Geometry check sheet. Reference: the model listing, model coordinates, mm. Face numbers are marked on the shaded views. Give positions to 0.01 mm unless a question says otherwise; leave off trailing zeros. Write each loop counter-clockwise with the first axis right and the second up, starting at its lowest first coordinate (ties: lowest second). Pieces come first, ordered by that corner, then holes. Notation, with made-up numbers: (-24.5, 32.25) -> (9.5, 32.25) arc R29 cw to (9.5, 71.25) -> close; hole circle Ø9 at (44.5, 72). An arc over 180 degrees is marked (long way). Use a Markdown table: item, result. Add a question column.
Autodesk Inventor part; units mm, degrees
ref_plane "YZ Plane" through (0, 0, 0) normal (1, 0, 0) x (0, 1, 0)
ref_plane "XZ Plane" through (0, 0, 0) normal (0, 1, 0) x (-1, 0, 0)
ref_plane "XY Plane" through (0, 0, 0) normal (0, 0, 1) x (1, 0, 0)
sketch "スケッチ1" plane through (0, 0, 0) normal (0, 0, 1) x (1, 0, 0)
  line L0 (-101.5, 48) -> (108.5, 48)
  circle A0 centre (111.885, -19) radius 4
  circle A1 centre (171.8807, -19.7195) radius 4
  circle A2 centre (111.885, -19) radius 7
  circle A3 centre (171.8807, -19.7195) radius 7
  line L1 (171.8807, -19.7195) -> (111.885, -19) construction
  line L2 (171.9647, -12.72) -> (111.969, -12.0005)
  line L3 (111.8011, -25.9995) -> (171.7968, -26.719)
  arc A4 (171.7968, -26.719) -> (171.9647, -12.72) centre (171.8807, -19.7195) ccw
  arc A5 (111.969, -12.0005) -> (111.8011, -25.9995) centre (111.885, -19) ccw
  line L4 (173.7961, -12.9866) -> (250.1906, -34.7195)
  circle A6 centre (241.9819, -63.5746) radius 30
  line L5 (268.18, -78.1916) -> (221.9512, -41.2414)
  line L6 (221.9512, -41.2414) -> (169.9654, -26.4523)
  line L7 (271.9819, -113.1361) -> (271.9819, -54.8199)
  line L8 (111.885, -19) -> (111.885, 41) construction
  line L9 (118.885, -19) -> (118.885, 41)
  line L10 (104.885, 41) -> (104.885, -19)
  arc A7 (104.885, -19) -> (118.885, -19) centre (111.885, -19) ccw
  arc A8 (118.885, 41) -> (104.885, 41) centre (111.885, 41) ccw
  circle A9 centre (29.4318, 47.238) radius 30
  line L11 (113.3193, 34.1485) -> (35.5787, 17.8745)
  line L12 (-0.5585, 48) -> (57.5489, 36.7771)
  line L13 (57.5489, 36.7771) -> (110.4508, 47.8515)
  circle A10 centre (113.5, -20) radius 68
  line L14 (321.9635, -82.9551) -> (60.2705, 100.2843)
  line L15 (259.1892, -39) -> (111.885, -19)
  arc A11 (93.5924, -27.1048) -> (135.371, -5.9244) centre (95.0604, 21.7941) ccw
  arc A12 (135.371, -5.9244) -> (135.8476, -3.6716) centre (132.899, -4.2246) ccw
  arc A13 (135.8476, -3.6716) -> (83.1833, 18.5565) centre (102.1579, -9.9896) ccw
  line L16 (111.885, -19) -> (112.6892, 40.9946) construction
  line L17 (118.8844, -19.0938) -> (119.6886, 40.9008)
  line L18 (105.6898, 41.0884) -> (104.8857, -18.9062)
  arc A14 (104.8857, -18.9062) -> (118.8844, -19.0938) centre (111.885, -19) ccw
  arc A15 (119.6886, 40.9008) -> (105.6898, 41.0884) centre (112.6892, 40.9946) ccw
  line L19 (164.9949, 48) -> (164.9949, 26)
  line L20 (164.9949, 26) -> (327.4949, -102)
  circle A16 centre (116.2926, -40) radius 68
  circle A17 centre (-98.885, 0) radius 67.5
  line L21 (321.3633, -8.501) -> (-152.6681, 78.4982)
  line L22 (104.8897, -3) -> (104.8897, 0)
  line L23 (104.8897, -3) -> (72.0656, -3)
  line L24 (72.0656, 0) -> (104.8897, 0)
  circle A18 centre (83.3769, -17.5) radius 13.85
  line L25 (178.7705, -28.9572) -> (174.2123, -32.8589)
  line L26 (174.2123, -32.8589) -> (164.8807, -30.2042)
  line L27 (164.8807, -30.2042) -> (164.8807, -19.7195)
  line L28 (169.9654, -26.4523) -> (168.5972, -31.2615)
  line L29 (168.5972, -31.2615) -> (164.8807, -26.636)
  line L30 (178.8802, -19.8034) -> (178.6547, -38.6089)
  line L31 (165.0125, -21.0715) -> (158.1724, 13.6763)
  circle A19 centre (171.8807, -19.7195) radius 7.5
  point P0 (0, 0)
  point P1 (141.8829, -19.3597)
  point P2 (111.885, 11)
  point P3 (105.885, 0)
  point P4 (105.885, 0)
  point P5 (23.7328, -42.729)
  point P6 (112.2871, 10.9973)
  point P7 (169.2723, -12.6877)
  point P8 (163.3482, -12.6166)
  point P9 (164.4925, -18.4296)
  point P10 (172.5552, -27.1891)
  point P11 (178.8479, -22.4958)
  dimension "d0" = 8
  dimension "d1" = 8
  dimension "d2" = 3
  dimension "d3" = 3
  dimension "d4" = 60
  dimension "d5" = 14
  dimension "d6" = 14
  dimension "d7" = 60
  dimension "d8" = 14
  dimension "d9" = 60
  dimension "d10" = 14
  dimension "d11" = 6
  dimension "d12" = 35
  dimension "d13" = 13.271
  dimension "d14" = 14
  dimension "d15" = 20
  dimension "d16" = 15
  dimension "d17" = 22
  dimension "d18" = 150
  dimension "d19" = 162.5
  dimension "d20" = 0
  dimension "d21" = 136
  dimension "d22" = 136
  dimension "d23" = 135
  dimension "d24" = 38.227
  dimension "d25" = 18
  dimension "d27" = 5
  dimension "d28" = 6
  dimension "d30" = 101.823
  dimension "d31" = 101.823
  dimension "d32" = 0.5
extrude "押し出し1" add sketch "スケッチ1" against normal blind 5 contours L25 L26 L28 A19 L15 L6 | L6 L15 L30 | L15 A19 L6 | L6 A19 L30 L15 | A19 L15 L28 L3 L6 | L6 L3 A3 L30 A19 | A19 L28 L15 | L29 L3 L15 A19 L28 | L26 L27 L29 | A2 A11 | L6 A3 L3 | L3 L28 L6 | L28 A19 L15 | L15 A19 L3 L28 | L27 L15 L3 | L3 A2 A11 L15 L27 | A3 | L9 A2 L2 | L2 L17 L9 | L3 A19 L27 L31 A3 L28 | L15 L3 A19 | A2 A11 | L15 L27 A19 L3 | L15 A11 L2 L31 A19 L27 | A19 L31 L2 | L2 A3 L27 L31 A19 | L2 A11 L15 A2 L17 | L31 L27 A3 | A2 L15 A11 | A19 L31 L27 | A0 | A1
extrude "押し出し2" cut sketch "スケッチ1" against normal blind 2.55 contours L6 L15 L30 | L6 A19 L30 L15 | A19 L15 L28 L3 L6 | L6 L3 A3 L30 A19 | A19 L28 L15 | L30 A3 L4 A19 | L6 A3 L3 | L3 L28 L6 | L28 A19 L15 | L15 A19 L3 L28 | A3 | L4 A3 L2 A19 | L3 A19 L27 L31 A3 L28 | A19 L31 L2 | L2 A3 L27 L31 A19 | L31 L27 A3 | A19 L31 L27 | A1
hole "穴1" at (105.885, 0, 0) at (23.7328, -42.729, 0) at (116.2926, -40, 0) at (-98.885, 0, 0) at (171.8807, -19.7195, 0) direction (0, 0, -1) diameter 3 depth 12 tip angle 118
sketch "スケッチ2" plane through (0, 0, 0) normal (0, 0, 1) x (1, 0, 0)
  line L0 (163.3482, -12.6166) -> (164.4925, -18.4296)
  arc A0 (164.4925, -18.4296) -> (172.5552, -27.1891) centre (171.8807, -19.7195) ccw
  line L1 (172.5552, -27.1891) -> (178.7705, -28.9572)
  line L2 (178.7705, -28.9572) -> (174.2123, -32.8589)
  line L3 (174.2123, -32.8589) -> (164.8807, -30.2042)
  line L4 (164.8807, -30.2042) -> (164.8807, -26.636)
  line L5 (164.8807, -26.636) -> (111.8011, -25.9995)
  arc A1 (111.969, -12.0005) -> (111.8011, -25.9995) centre (111.885, -19) ccw
  line L6 (111.969, -12.0005) -> (163.3482, -12.6166)
  circle A2 centre (171.8807, -19.7195) radius 7.5
  circle A3 centre (171.8807, -19.7195) radius 12.5
  point P0 (0, 0)
  point P1 (161.4414, -26.5948)
  point P2 (164.8807, -30.0756)
  point P3 (165.2308, -30.3038)
  point P4 (171.9637, -32.2192)
  dimension "d44" = 5
extrude "押し出し3" add sketch "スケッチ2" against normal blind 5 contours L5 L4 A3 | A3 L3
sketch "スケッチ3" plane through (0, 0, 0) normal (0, 0, 1) x (1, 0, 0)
  line L0 (163.3482, -12.6166) -> (164.4925, -18.4296)
  arc A0 (164.4925, -18.4296) -> (172.5552, -27.1891) centre (171.8807, -19.7195) ccw
  line L1 (172.5552, -27.1891) -> (178.7705, -28.9572)
  line L2 (178.7705, -28.9572) -> (174.2123, -32.8589)
  line L3 (174.2123, -32.8589) -> (171.9637, -32.2192)
  arc A1 (165.2308, -30.3038) -> (171.9637, -32.2192) centre (171.8807, -19.7195) ccw
  line L4 (165.2308, -30.3038) -> (164.8807, -30.2042)
  line L5 (164.8807, -30.2042) -> (164.8807, -30.0756)
  arc A2 (161.4414, -26.5948) -> (164.8807, -30.0756) centre (171.8807, -19.7195) ccw
  line L6 (161.4414, -26.5948) -> (111.8011, -25.9995)
  arc A3 (111.969, -12.0005) -> (111.8011, -25.9995) centre (111.885, -19) ccw
  line L7 (111.969, -12.0005) -> (163.3482, -12.6166)
  circle A4 centre (171.8807, -19.7195) radius 12.5
  point P0 (0, 0)
  point P1 (165.2308, -30.3038)
extrude "押し出し4" cut sketch "スケッチ3" against normal blind 10 contours A4 L4 L5
hole "穴2" at (105.885, 0, 0) at (111.885, -19, 0) direction (0, 0, -1) diameter 8.05 depth 12 tip angle 118
sketch "スケッチ4" plane through (0, 0, 0) normal (0, 0, 1) x (1, 0, 0)
  circle A0 centre (111.885, -19) radius 4.025
  line L0 (163.3482, -12.6166) -> (164.4925, -18.4296)
  arc A1 (164.4925, -18.4296) -> (172.5552, -27.1891) centre (171.8807, -19.7195) ccw
  line L1 (172.5552, -27.1891) -> (178.7705, -28.9572)
  line L2 (178.7705, -28.9572) -> (174.2123, -32.8589)
  line L3 (174.2123, -32.8589) -> (171.9637, -32.2192)
  arc A2 (161.4414, -26.5948) -> (171.9637, -32.2192) centre (171.8807, -19.7195) ccw
  line L4 (161.4414, -26.5948) -> (111.8011, -25.9995)
  arc A3 (111.969, -12.0005) -> (111.8011, -25.9995) centre (111.885, -19) ccw
  line L5 (111.969, -12.0005) -> (163.3482, -12.6166)
  arc A4 (164.4925, -18.4296) -> (172.5552, -27.1891) centre (171.8807, -19.7195) ccw
  circle A5 centre (171.8807, -19.7195) radius 7.5
  circle A6 centre (171.8807, -19.7195) radius 9
  line L6 (178.7705, -28.9572) -> (172.5552, -27.1891)
  line L7 (164.4925, -18.4296) -> (163.3482, -12.6166)
  circle A7 centre (111.885, -19) radius 9
  point P0 (0, 0)
  point P1 (175.4063, -28.0002)
  point P2 (163.9203, -15.5231)
  point P3 (163.92, -15.5211)
  point P4 (175.4063, -28.0002)
  dimension "d56" = 15
  dimension "d57" = 1.5
  dimension "d58" = 18
extrude "押し出し5" add sketch "スケッチ4" against normal blind 5 contours A7 L4 A3 L5 | L5 A3 L4 A7
extrude "押し出し6" cut sketch "スケッチ4" against normal blind 2.55 contours L0 A1 L1 A6
sketch "スケッチ5" plane through (0, 0, 0) normal (0, 0, 1) x (1, 0, 0)
  arc A0 (117.6254, -12.0683) -> (117.4576, -26.0673) centre (111.885, -19) ccw
  line L0 (117.6254, -12.0683) -> (163.3482, -12.6166)
  line L1 (163.3482, -12.6166) -> (163.92, -15.5211)
  arc A1 (163.92, -15.5211) -> (175.4063, -28.0002) centre (171.8807, -19.7195) ccw
  line L2 (175.4063, -28.0002) -> (178.7705, -28.9572)
  line L3 (178.7705, -28.9572) -> (174.2123, -32.8589)
  line L4 (174.2123, -32.8589) -> (171.9637, -32.2192)
  arc A2 (161.4414, -26.5948) -> (171.9637, -32.2192) centre (171.8807, -19.7195) ccw
  line L5 (161.4414, -26.5948) -> (117.4576, -26.0673)
  circle A3 centre (111.885, -19) radius 4.025
  circle A4 centre (111.885, -19) radius 6
  point P0 (0, 0)
  dimension "d63" = 12
extrude "押し出し7" cut sketch "スケッチ5" against normal blind 1 contours A4
sketch "スケッチ6" plane through (0, 0, 0) normal (0, 0, 1) x (1, 0, 0)
  circle A0 centre (111.885, -19) radius 6
  arc A1 (161.4414, -26.5948) -> (171.9637, -32.2192) centre (171.8807, -19.7195) ccw
  line L0 (161.4414, -26.5948) -> (117.4576, -26.0673)
  arc A2 (117.6254, -12.0683) -> (117.4576, -26.0673) centre (111.885, -19) ccw
  line L1 (117.6254, -12.0683) -> (163.3482, -12.6166)
  line L2 (163.3482, -12.6166) -> (163.92, -15.5211)
  arc A3 (163.92, -15.5211) -> (175.4063, -28.0002) centre (171.8807, -19.7195) ccw
  line L3 (175.4063, -28.0002) -> (178.7705, -28.9572)
  line L4 (178.7705, -28.9572) -> (174.2123, -32.8589)
  line L5 (174.2123, -32.8589) -> (171.9637, -32.2192)
  circle A4 centre (171.8807, -19.7195) radius 1.5
  circle A5 centre (171.8807, -19.7195) radius 3
  point P0 (0, 0)
  dimension "d66" = 6
extrude "押し出し8" cut sketch "スケッチ6" against normal blind 3 contours A5
equation "\"d9\" = d7"
equation "\"d31\" = d30"
properties part number "後ろウィング中間"
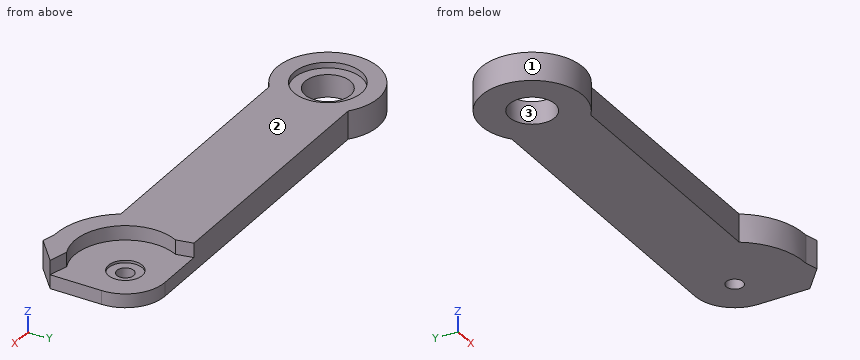
1) Material ranges on probe 1 along X at (y, z) = (-19, -3.5) (3 decimals); probe 2 along X at (y, z) = (-20, -4.1); probe 3 along X at (y, z) = (-19, -2.5) (1 decimal), recorded low to high. Write a range as [from, to].
2) Sectioned sample at D-D, the plane y = -14. Enter the section's corners in (x, z), and give its area (3 significant figures).
3) Gauge pin test, flat ends, axial feed: P1, Ø9.5, axis at x = 171.88, y = -19.72, coming from the +Z side; P2, Ø3, axis at x = 153.5, z = -4.5, coming from the +Y side; P3, Ø2, axis at x = 127.5, z = -2, coming from the +Y side. Record the tip position at first contact, or that the pin passes through.
4) Sectioned sample at B-B, the plane x = 109.5. Enter the section's corners in (y, z).
5) Sectioned sample at A-A, the plane y = -19. Count the separate pieces of the cut face and the enclosed holes in it, and give its area (3 significant figures).
6) Draft check along Y on the marked faces 1, 2 and 3. Enter one of: +Y half, -Y half, draft (parallel to the pull), parting line (faces both ways), or undercut.
Check values:
| question | item | result |
|---|---|---|
| 1 | probe 1 | [102.885, 107.86], [115.91, 170.565], [173.197, 178.844] |
| 1 | probe 2 | [102.94, 107.99], [115.78, 170.41], [173.35, 178.88] |
| 1 | probe 3 | [102.9, 107.9], [115.9, 162.9] |
| 2 | outline | (104.4, -5) -> (175.92, -5) -> (175.92, -2.55) -> (163.62, -2.55) -> (163.62, 0) -> (115.2, 0) -> (115.2, -1) -> (108.57, -1) -> (108.57, 0) -> (104.4, 0) -> close |
| 2 | area | 320 mm² |
| 3 | P1 | z = -2.55 |
| 3 | P2 | y = -12.48 |
| 3 | P3 | y = -12.17 |
| 4 | outline | (-27.68, -5) -> (-22.24, -5) -> (-22.24, -1) -> (-24.51, -1) -> (-24.51, 0) -> (-27.68, 0) -> close; (-15.76, -5) -> (-10.32, -5) -> (-10.32, 0) -> (-13.49, 0) -> (-13.49, -1) -> (-15.76, -1) -> close |
| 5 | separate pieces | 3 |
| 5 | enclosed holes | 0 |
| 5 | area | 287 mm² |
| 6 | face 1 | parting line |
| 6 | face 2 | draft |
| 6 | face 3 | undercut |
